Job drawing, mm, ordinate dimensions from the low corner. One solid piece. A direction names the side the tool comes from. Coordinates: 2 decimals unless noted, no trailing zeros. Loops run counter-clockwise (first coordinate to the right, second up) from the corner with the lowest first, then second, coordinate; pieces in that order, holes last. Notation, with made-up numbers: (-1.5, 68.25) -> (49.5, 68.25) arc R21 cw to (49.5, 85.25) -> close; hole circle Ø1 at (-16.75, 45.5). An arc over 180 degrees is marked (long way). Use one line per item in the form item = value. Start each with the question number.
(1) Band-saw the part on A-A on x = 30.16. Give the cut face in (y, z), then the cut area to 3 significant figures.
(2) Band-saw the part on C-C on y = 9. Give the cut face in (x, z).
(3) Drill centre lines: L1, parallel to Z at x = 30, y = 6; L2, parallel to X at y = 11, z = 13.65; L3, parallel to Z at x = 25, y = 38. Where is each one in solid material? Low to high. Write a range as [from, to].
(4) 3-axis set-ups, long thin cutter, end or side, ignore diameter. For the marked faces 1, 2 and 3: which of +Z, -Z, +X, -X, +Y, -Y reach the whole face in a straight line?
(5) Pin check, flat tips, straight feed: P1, Ø6.5, axis at y = 17.5, z = 23.5, coming from the -X side; P2, Ø11, axis at x = 20, z = 17, coming from the +Y side. Stop position of each tip, or through.
(6) Band-saw the part on D-D on x = 24. Give the cut face in (y, z).
(7) Band-saw the part on B-B on z = 26.35. Give the cut face in (x, y).
(8) Mould opens along Z. For the marked faces 4, 5, 6 and 7 say: +Z half, -Z half, draft (parallel to the pull), parting line (faces both ways), or undercut.
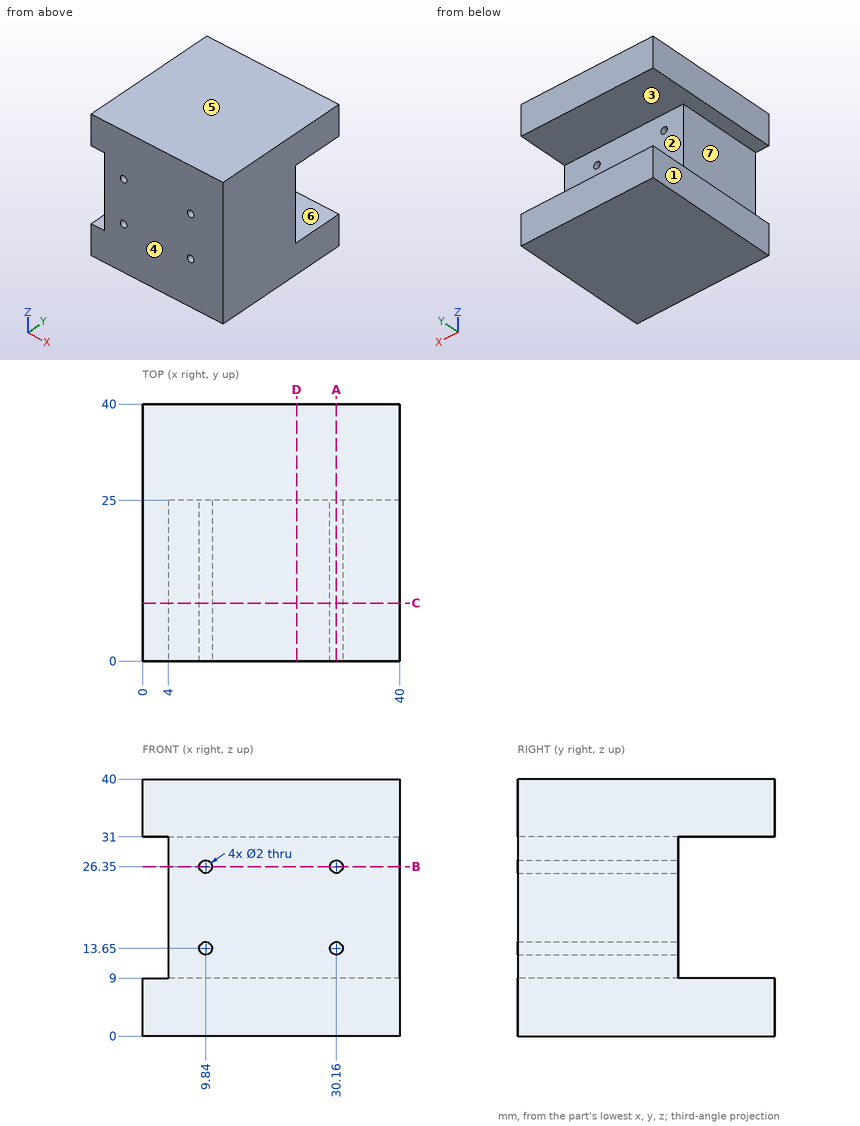
A:
q1.outline = (0, 0) -> (40, 0) -> (40, 9) -> (25, 9) -> (25, 12.65) -> (0, 12.65) -> close; (0, 14.65) -> (25, 14.65) -> (25, 25.35) -> (0, 25.35) -> close; (0, 27.35) -> (25, 27.35) -> (25, 31) -> (40, 31) -> (40, 40) -> (0, 40) -> close
q1.area = 1,170 mm²
q2.outline = (0, 0) -> (40, 0) -> (40, 40) -> (0, 40) -> (0, 31) -> (4, 31) -> (4, 9) -> (0, 9) -> close; hole circle Ø2 at (9.84, 13.65); hole circle Ø2 at (9.84, 26.35); hole circle Ø2 at (30.16, 13.65); hole circle Ø2 at (30.16, 26.35)
q3.L1 = [0, 12.66], [14.64, 25.36], [27.34, 40]
q3.L2 = [4, 8.84], [10.84, 29.16], [31.16, 40]
q3.L3 = [0, 9], [31, 40]
q4.face_1 = +Z, -Z, -X, +Y, -Y
q4.face_2 = +X, -X, +Y
q4.face_3 = -X, +Y
q5.P1 = 4
q5.P2 = 25
q6.outline = (0, 0) -> (40, 0) -> (40, 9) -> (25, 9) -> (25, 31) -> (40, 31) -> (40, 40) -> (0, 40) -> close
q7.outline = (4, 0) -> (8.84, 0) -> (8.84, 25) -> (4, 25) -> close; (10.84, 0) -> (29.16, 0) -> (29.16, 25) -> (10.84, 25) -> close; (31.16, 0) -> (40, 0) -> (40, 25) -> (31.16, 25) -> close
q8.face_4 = draft
q8.face_5 = +Z half
q8.face_6 = undercut
q8.face_7 = undercut
